```python
from build123d import *

# Parameters (mm, degrees)
SKETCH1_R                 = 1.651
BOSS_EXTRUDE2_DEPTH       = 5.3975
SKETCH2_R                 = 1.143
CUT_EXTRUDE1_DEPTH        = 6.3975
SKETCH3_R                 = 12.1285
CUT_EXTRUDE2_DEPTH        = 6.3975
SKETCH4_W                 = 28.562713242
SKETCH4_H                 = 11.677503754
BOSS_EXTRUDE3_DEPTH       = 5.3975
SKETCH5_W                 = 216.7214489
SKETCH5_H                 = 130.569220634
CUT_EXTRUDE4_DEPTH        = 6.3975
SKETCH6_R                 = 38.1
CUT_EXTRUDE5_DEPTH        = 60.96
FILLET1_R                 = 6.35
FILLET2_R                 = 6.35
SKETCH102_W               = 8.89
SKETCH102_H               = 8.89
CUT_EXTRUDE101_DEPTH      = 6.3975001
SKETCH105_R               = 5
CUT_EXTRUDE104_DEPTH      = 10
SKETCH106_R               = 3.175
CUT_EXTRUDE105_DEPTH      = 103.378
CUT_EXTRUDE105_DEPTH_BACK = 1
SKETCH158_R               = 1.651
CUT_EXTRUDE157_DEPTH      = 97.79


with BuildPart() as part:
    # Sketch1 → Boss-Extrude2 (new body)
    with BuildSketch(Plane.XY):
        with BuildLine():
            Line((-64.964441474, 37.338), (-54.550441474, 37.338))
            Line((-54.550441474, 37.338), (-54.550441474, -37.338))
            Line((-54.550441474, -37.338), (-64.964441474, -37.338))
            ThreePointArc((-64.964441474, -37.338), (0, -74.93), (64.964441474, -37.338))
            Line((64.964441474, -37.338), (54.550441474, -37.338))
            Line((54.550441474, -37.338), (54.550441474, 37.338))
            Line((54.550441474, 37.338), (64.964441474, 37.338))
            ThreePointArc((64.964441474, 37.338), (0, 74.93), (-64.964441474, 37.338))
        make_face()
        with Locations((-46.482, 11.049)):
            Circle(SKETCH1_R, mode=Mode.SUBTRACT)
        with Locations((-21.083270032, 10.795)):
            Circle(SKETCH1_R, mode=Mode.SUBTRACT)
        with Locations((-21.083270032, -10.795)):
            Circle(SKETCH1_R, mode=Mode.SUBTRACT)
        with Locations((-46.482, -11.049)):
            Circle(SKETCH1_R, mode=Mode.SUBTRACT)
        with Locations((46.482, -11.049)):
            Circle(SKETCH1_R, mode=Mode.SUBTRACT)
        with Locations((21.083270032, -10.795)):
            Circle(SKETCH1_R, mode=Mode.SUBTRACT)
        with Locations((21.083270032, 10.795)):
            Circle(SKETCH1_R, mode=Mode.SUBTRACT)
        with Locations((46.482, 11.049)):
            Circle(SKETCH1_R, mode=Mode.SUBTRACT)
    extrude(amount=BOSS_EXTRUDE2_DEPTH)

    # Sketch2 → Cut-Extrude1 (cut, through all)
    with BuildSketch(Plane.XY.offset(5.3975)):
        with Locations((-6.731, 62.23)):
            Circle(SKETCH2_R)
        with Locations((6.731, 62.23)):
            Circle(SKETCH2_R)
    extrude(amount=-CUT_EXTRUDE1_DEPTH, mode=Mode.SUBTRACT)

    # Sketch3 → Cut-Extrude2 (cut, through all)
    with BuildSketch(Plane(origin=(0, 0, 0), x_dir=(-1, 0, 0), z_dir=(0, 0, -1))):
        with Locations((-43.105229381, -43.105229381)):
            Circle(SKETCH3_R)
        with Locations((14.224, -34.29)):
            Circle(SKETCH3_R)
        with Locations((14.224, 34.29)):
            Circle(SKETCH3_R)
        with Locations((-43.105229381, 43.105229381)):
            Circle(SKETCH3_R)
        with Locations((43.105229381, 43.105229381)):
            Circle(SKETCH3_R)
        with Locations((-14.224, 34.29)):
            Circle(SKETCH3_R)
        with Locations((-14.224, -34.29)):
            Circle(SKETCH3_R)
        with Locations((43.105229381, -43.105229381)):
            Circle(SKETCH3_R)
    extrude(amount=-CUT_EXTRUDE2_DEPTH, mode=Mode.SUBTRACT)

    # Sketch4 → Boss-Extrude3 (add)
    with BuildSketch(Plane(origin=(0, 0, 0), x_dir=(-1, 0, 0), z_dir=(0, 0, -1))):
        with Locations((-1.488809975, 62.152540216)):
            Rectangle(SKETCH4_W, SKETCH4_H)
    extrude(amount=-BOSS_EXTRUDE3_DEPTH)

    # Sketch5 → Cut-Extrude4 (cut, through all)
    with BuildSketch(Plane(origin=(0, 0, 0), x_dir=(-1, 0, 0), z_dir=(0, 0, -1))):
        with Locations((23.316688373, 48.139610317)):
            Rectangle(SKETCH5_W, SKETCH5_H)
    extrude(amount=-CUT_EXTRUDE4_DEPTH, mode=Mode.SUBTRACT)

    # Sketch6 → Cut-Extrude5 (cut)
    with BuildSketch(Plane(origin=(0, 0, 0), x_dir=(-1, 0, 0), z_dir=(0, 0, -1))):
        with Locations((0, -86.312058398)):
            Circle(SKETCH6_R)
    extrude(amount=-CUT_EXTRUDE5_DEPTH, mode=Mode.SUBTRACT)

    # Fillet1
    fillet1_edges = [part.edges().sort_by_distance(p)[0] for p in [
        (-33.000960548, -67.271401821, 2.69875),
    ]]
    fillet(fillet1_edges, radius=FILLET1_R)

    # Fillet2
    fillet2_edges = [part.edges().sort_by_distance(p)[0] for p in [
        (33.000960548, -67.271401821, 2.69875),
    ]]
    fillet(fillet2_edges, radius=FILLET2_R)

    # Sketch102 → Cut-Extrude101 (cut, through all)
    with BuildSketch(Plane(origin=(0, 0, 0), x_dir=(-1, 0, 0), z_dir=(0, 0, -1))):
        with Locations((-33.605441474, -21.59)):
            Rectangle(SKETCH102_W, SKETCH102_H)
        with Locations((33.605441474, -21.59)):
            Rectangle(SKETCH102_W, SKETCH102_H)
    extrude(amount=-CUT_EXTRUDE101_DEPTH, mode=Mode.SUBTRACT)

    # Sketch105 → Cut-Extrude104 (cut)
    with BuildSketch(Plane(origin=(0, 0, 0), x_dir=(-1, 0, 0), z_dir=(0, 0, -1))):
        with Locations((-12.7, -15.24)):
            Circle(SKETCH105_R)
        with Locations((12.7, -15.24)):
            Circle(SKETCH105_R)
    extrude(amount=-CUT_EXTRUDE104_DEPTH, mode=Mode.SUBTRACT)

    # Sketch106 → Cut-Extrude105 (cut, two sides)
    with BuildSketch(Plane(origin=(30.092005081, 4.08352975, 22.2885), x_dir=(-1, 0, 0), z_dir=(0, 0, -1))) as cut_extrude105_sk:
        with Locations((73.272005081, -29.48352975)):
            Circle(SKETCH106_R)
        with Locations((30.092005081, -29.48352975)):
            Circle(SKETCH106_R)
        with Locations((-13.087994919, -29.48352975)):
            Circle(SKETCH106_R)
    extrude(amount=CUT_EXTRUDE105_DEPTH, mode=Mode.SUBTRACT)
    extrude(cut_extrude105_sk.sketch, amount=-CUT_EXTRUDE105_DEPTH_BACK, mode=Mode.SUBTRACT)

    # Sketch158 → Cut-Extrude157 (cut)
    with BuildSketch(Plane(origin=(30.092005081, 4.08352975, -24.638), x_dir=(-1, 0, 0), z_dir=(0, 0, -1))):
        with Locations((4.154396091, -49.728759131)):
            Circle(SKETCH158_R)
        with Locations((56.02961407, -49.728759131)):
            Circle(SKETCH158_R)
    extrude(amount=-CUT_EXTRUDE157_DEPTH, mode=Mode.SUBTRACT)


solid = part.part
```
Geometry: final body of the model. Coordinates: model frame, mm. A direction names the side the tool comes from. Round coordinates to 2 decimals unless told otherwise and drop trailing zeros. Order: outer loops, then holes, each group sorted by start corner. A loop starts at its lowest first (then second) coordinate and runs counter-clockwise, first axis right, second up. Notation, with made-up numbers: (43, -38) - (54, -38) arc R9 ccw to (54, -29) - close; hole circle Ø11 at (-30.75, 43.25). An arc over 180 degrees is marked (long way). Write item = value, one per line. Start each with the question number.
Q1. Pull-direction query (Y, two-part tool) for faces 1 (the flat face through (-34, -26.035, 3)), 2 (the cylindrical face through (53.178, -52.788, 2.661)), 3 (the cylindrical face through (26.296, -47.257, 2.661)); classes: +Y half, -Y half, draft (parallel to the pull), parting line (faces both ways), or undercut.
Q2. Ray query, line 1 (X direction, y = -20.5, z = 4.85); line 2 (Y direction, x = -46, z = 0.85) (3 decimals); line 3 (X direction, y = -47.5, z = 4.75). Return the intervals inside material, ascending. Write a range as from..to.
Q3. Cut plane D-D on y = -61. Return the cut outline in (x, z).
Q4. Cut plane A-A on x = 21. Return the cut outline in (y, z) (1 decimal), and give its area (3 significant figures).
Q5. Access query for faces 4 (the flat face through (54.55, -27, 3)), 5 (the flat face through (29.16, -22, 3)), 6 (the flat face through (-60, -37.338, 3)). Directions: +Z, -Z, +X, -X, +Y, -Y. A direction counts if a zero-diameter tool reaches every point of the face in a straight line with its end or side. Return the directions, or none.
Q6. Cut plane C-C on y = -53.5. Return the cut outline in (x, z).
Q7. Cut plane B-B on y = -34.29. Return the cut outline in (x, z).
Q8. Pin query (flat end, axial travel): pin 1 (1.6 mm diameter, centred on y = -31, z = 4, fed in from +X); pin 2 (1 mm diameter, centred on y = -26, z = 1.5, fed in from -X); pin 3 (1.6 mm diameter, centred on x = 33, z = 2.5, fed in from +Y) (3 decimals); pin 4 (3 mm diameter, centred on x = -39, y = -35.5, fed in from +Z). Return the tip coordinate at first contact, or that it passes through.
Outcome:
q1.face_1 = +Y half
q1.face_2 = -Y half
q1.face_3 = undercut
q2.line_1 = -54.55..-38.05, -29.16..29.16, 38.05..54.55
q2.line_2 = -59.148..-54.883, -31.327..-26.859, -23.941..-17.145
q2.line_3 = -57.95..-54.41, -31.8..31.8, 54.41..57.95
q3.outline = (-43.51, 0) - (-28.48, 0) - (-28.48, 5.4) - (-43.51, 5.4) - close; (28.48, 0) - (43.51, 0) - (43.51, 5.4) - (28.48, 5.4) - close
q4.outline = (-54.5, 0) - (-44.3, 0) - (-44.3, 5.4) - (-54.5, 5.4) - close; (-24.2, 0) - (-17.1, 0) - (-17.1, 5.4) - (-24.2, 5.4) - close
q4.area = 93.2 mm^2
q5.face_4 = +Z, -Z, +X, +Y
q5.face_5 = +Z, -Z, +Y
q5.face_6 = +Z, -Z, -X, +Y
q6.outline = (-52.46, 0) - (-49.35, 0) - (-49.35, 5.4) - (-52.46, 5.4) - close; (-36.86, 0) - (-19.36, 0) - (-19.36, 5.4) - (-36.86, 5.4) - close; (19.36, 0) - (36.86, 0) - (36.86, 5.4) - (19.36, 5.4) - close; (49.35, 0) - (52.46, 0) - (52.46, 5.4) - (49.35, 5.4) - close
q7.outline = (-54.55, 0) - (-51.44, 0) - (-51.44, 5.4) - (-54.55, 5.4) - close; (-34.78, 0) - (-26.35, 0) - (-26.35, 5.4) - (-34.78, 5.4) - close; (-2.1, 0) - (2.1, 0) - (2.1, 5.4) - (-2.1, 5.4) - close; (26.35, 0) - (34.78, 0) - (34.78, 5.4) - (26.35, 5.4) - close; (51.44, 0) - (54.55, 0) - (54.55, 5.4) - (51.44, 5.4) - close
q8.pin_1 = 54.55
q8.pin_2 = -54.55
q8.pin_3 = -26.035
q8.pin_4 = through
